Verification items for the finished model (mm, model axes). A direction names the side the tool comes from. Round coordinates to 2 decimals unless told otherwise and drop trailing zeros. Loops run counter-clockwise (first coordinate to the right, second up) from the corner with the lowest first, then second, coordinate; pieces in that order, holes last. Notation, with made-up numbers: (-1.75, 23.25) - (51.25, 23.25) arc R14 cw to (51.25, 34.25) - close; hole circle Ø8 at (31.5, -39). An arc over 180 degrees is marked (long way). Use a Markdown table: item, result. Add a question column.
```python
from build123d import *

# Parameters (mm, degrees)
F0_W     = 114.8236654699
F0_H     = 108.2134023309
F1_DEPTH = 104
F2_W     = 12.52374053
F2_H     = 20.7482948899
F2_W_2   = 12.2485402972
F2_H_2   = 20.5613672733
F2_W_3   = 11.7760580033
F2_W_4   = 13.0845084786
F3_DEPTH = 114.8246654699
F4_W     = 60
F4_H     = 17.0350422454
F4_W_2   = 9
F4_H_2   = 18.0536039271
F4_H_3   = 18.2386368836
F4_H_4   = 17.2398763835
F4_W_3   = 12
F4_H_5   = 23.2148324465
F5_DEPTH = 25
F6_R     = 3.9918066597
F6_R_2   = 3.9469258839
F6_R_3   = 3.3313946803
F6_R_4   = 3.8357142578
F6_R_5   = 3.700614932
F7_DEPTH = 114.8246654699
F8_R     = 5.3166490127
F9_DEPTH = 15.7


with BuildPart() as f1:
    # F0 (on Top) → F1 (new body)
    with BuildSketch(Plane.XY):
        with Locations((13.4518984705, 2.4405606091)):
            Rectangle(F0_W, F0_H)
    extrude(amount=F1_DEPTH)

    # F2 (on face) → F3 (cut, through all)
    with BuildSketch(Plane.YZ.offset(70.8637312055)):
        with Locations((-32.5295254588, 96.3900126517)):
            Rectangle(F2_W, F2_H)
        with Locations((-6.1242701486, 96.2965488434)):
            Rectangle(F2_W_2, F2_H_2)
        with Locations((16.6308367625, 96.3900126517)):
            Rectangle(F2_W_3, F2_H)
        with Locations((38.9679595828, 96.2965488434)):
            Rectangle(F2_W_4, F2_H_2)
    extrude(amount=-F3_DEPTH, mode=Mode.SUBTRACT)

    # F4 (on face) → F5 (cut)
    with BuildSketch(Plane.XY.offset(104)):
        with Locations((14.153456504, -45.1724111309)):
            Rectangle(F4_W, F4_H)
        with Locations((10.6519766077, -18.7213037212)):
            Rectangle(F4_W_2, F4_H_2)
        with Locations((-7.7669977982, 4.9567892806)):
            Rectangle(F4_W_2, F4_H_3)
        with Locations((12.4489111735, 26.4460458092)):
            Rectangle(F4_W, F4_H_4)
        with Locations((-13.255634157, 49.3767052152)):
            Rectangle(F4_W_3, F4_H_5)
    extrude(amount=-F5_DEPTH, mode=Mode.SUBTRACT)

    # F6 (on face) → F7 (cut, through all)
    with BuildSketch(Plane.YZ.offset(70.8637312055)):
        with Locations((-46.1977943778, 94.5423319936)):
            Circle(F6_R)
        with Locations((-20.0246851891, 94.7679579258)):
            Circle(F6_R_2)
        with Locations((5.0202719867, 95.4448506236)):
            Circle(F6_R_3)
        with Locations((50.3719523549, 94.9935913086)):
            Circle(F6_R_4)
        with Locations((27.132038027, 94.9935913086)):
            Circle(F6_R_5)
    extrude(amount=-F7_DEPTH, mode=Mode.SUBTRACT)

    # F8 (on face) → F9 (cut)
    with BuildSketch(Plane.YZ.offset(70.8637312055)):
        with Locations((-20.0246851891, 94.7679579258)):
            Circle(F8_R)
    extrude(amount=-F9_DEPTH, mode=Mode.SUBTRACT)


solid = f1.part
```
Q1. Thickness scan on line 1 along Z through (x, y) = (-18, 5); line 2 along Z through (x, y) = (-39, -26.5); line 3 along Z through (x, y) = (8.5, 7.5). Record the ranges inside material, lowest first.
Q2. Section check C-C on x = -29. Record the cut outline in (y, z), plus the area to 3 significant figures.
Q3. Section check D-D on x = 9. Record the cut outline in (y, z).
Q4. Go/stop test with flat-tipped pins: pin 1 Ø5.5 at (x, z) = (-6.5, 92.5) entering from -Y; pin 2 Ø6 at (x, y) = (12.5, 15.5) entering from +Z; pin 3 Ø4.5 at (x, y) = (9, -20) entering from +Z. Record where each tip stops, or that it passes through.
Q5. Set-up check for faces 3 (the face through (-8, 5, 79)), 4 (the face through (-13, 47, 79)), 5 (the face through (43, -12.249, 95)), 6 (the face through (13, 3, 0)): record each of +Z, -Z, +X, -X, +Y, -Y from which the full face is reachable in a straight line by a thin tool's end or side.
Q6. Release check for a two-part mould opening along X. For faces 1 (the face through (-13, 37.769, 83)), 2 (the face through (33, 5, 104)) record: +X half, -X half, draft (parallel to the pull), parting line (faces both ways), or undercut.
Q7. Section check B-B on y = 28.5. Record the cut outline in (x, z).
Q8. Section check A-A on z = 82. Record the cut outline in (x, y), plus the area to 3 significant figures.
Determined:
| question | item | result |
|---|---|---|
| 1 | line 1 | z = 0 to 92.11, 98.78 to 104 |
| 1 | line 2 | z = 0 to 86.02 |
| 1 | line 3 | z = 0 to 93.22, 97.67 to 104 |
| 2 | outline | (-51.67, 0) - (56.55, 0) - (56.55, 104) - (45.51, 104) - (45.51, 86.02) - (32.43, 86.02) - (32.43, 104) - (22.52, 104) - (22.52, 86.02) - (10.74, 86.02) - (10.74, 104) - (0, 104) - (0, 86.02) - (-12.25, 86.02) - (-12.25, 104) - (-26.27, 104) - (-26.27, 86.02) - (-38.79, 86.02) - (-38.79, 104) - (-51.67, 104) - close; hole circle Ø7.98 at (-46.2, 94.54); hole circle Ø7.89 at (-20.02, 94.77); hole circle Ø6.66 at (5.02, 95.44); hole circle Ø7.4 at (27.13, 94.99); hole circle Ø7.67 at (50.37, 94.99) |
| 2 | area | 10,100 mm² |
| 3 | outline | (-51.67, 0) - (56.55, 0) - (56.55, 104) - (45.51, 104) - (45.51, 86.02) - (35.07, 86.02) - (35.07, 79) - (17.83, 79) - (17.83, 86.02) - (10.74, 86.02) - (10.74, 104) - (0, 104) - (0, 86.02) - (-9.69, 86.02) - (-9.69, 79) - (-27.75, 79) - (-27.75, 86.02) - (-36.65, 86.02) - (-36.65, 79) - (-51.67, 79) - close; hole circle Ø6.66 at (5.02, 95.44); hole circle Ø7.67 at (50.37, 94.99) |
| 4 | pin 1 | stops at y = -26.27 |
| 4 | pin 2 | stops at z = 86.02 |
| 4 | pin 3 | stops at z = 79 |
| 5 | face 3 | +Z |
| 5 | face 4 | +Z, +Y |
| 5 | face 5 | +Z, +X, -X |
| 5 | face 6 | -Z, +X, -X, +Y, -Y |
| 6 | face 1 | undercut |
| 6 | face 2 | draft |
| 7 | outline | (-43.96, 0) - (70.86, 0) - (70.86, 91.56) - (42.45, 91.56) - (42.45, 79) - (-17.55, 79) - (-17.55, 91.56) - (-43.96, 91.56) - close; (-43.96, 98.43) - (-17.55, 98.43) - (-17.55, 104) - (-43.96, 104) - close; (42.45, 98.43) - (70.86, 98.43) - (70.86, 104) - (42.45, 104) - close |
| 8 | outline | (-43.96, -51.67) - (-15.85, -51.67) - (-15.85, -36.65) - (44.15, -36.65) - (44.15, -51.67) - (70.86, -51.67) - (70.86, 56.55) - (-7.26, 56.55) - (-7.26, 37.77) - (-19.26, 37.77) - (-19.26, 56.55) - (-43.96, 56.55) - close; hole (-17.55, 17.83) - (42.45, 17.83) - (42.45, 35.07) - (-17.55, 35.07) - close; hole (-12.27, -4.16) - (-3.27, -4.16) - (-3.27, 14.08) - (-12.27, 14.08) - close; hole (6.15, -27.75) - (15.15, -27.75) - (15.15, -9.69) - (6.15, -9.69) - close |
| 8 | area | 9,940 mm² |
